Check sheet for the modelled part. Datum: model origin and axes. Units: mm. A direction names the side the tool comes from. Round coordinates to 2 decimals unless told otherwise and drop trailing zeros. Write each loop counter-clockwise with the first axis right and the second up, starting at its lowest first coordinate (ties: lowest second). Pieces come first, ordered by that corner, then holes. Notation, with made-up numbers: M 53.5,-4.75 L 76.5,-4.75 A11 ccw 76.5,-0.75 Z; hole C 22,41.25 d11. An arc over 180 degrees is marked long. Answer in a Markdown table with one row per item.
```python
from build123d import *

# Parameters (mm, degrees)
F0_W     = 20
F0_H     = 10
F1_DEPTH = 5
F2_W     = 5
F2_H     = 30
F3_DEPTH = 30
F4_W     = 20
F4_H     = 5
F5_DEPTH = 5
F6_R     = 5
F7_DEPTH = 5


with BuildPart() as f1:
    # F0 (on Front) → F1 (new body)
    with BuildSketch(Plane.XZ):
        Polygon((0, 100), (0, 0), (142, 0), (142, 100), (50.6040596026, 100), (50.6040596026, 121.4291932336), (20, 100), align=None)
        with Locations((30.5, 25)):
            Rectangle(F0_W, F0_H, mode=Mode.SUBTRACT)
        with Locations((71, 25)):
            Rectangle(F0_W, F0_H, mode=Mode.SUBTRACT)
        with Locations((111.5, 25)):
            Rectangle(F0_W, F0_H, mode=Mode.SUBTRACT)
        with Locations((30.5, 75)):
            Rectangle(F0_W, F0_H, mode=Mode.SUBTRACT)
        with Locations((71, 75)):
            Rectangle(F0_W, F0_H, mode=Mode.SUBTRACT)
        with Locations((111.5, 75)):
            Rectangle(F0_W, F0_H, mode=Mode.SUBTRACT)
    extrude(amount=F1_DEPTH)

    # F2 (on face) → F3 (join)
    with BuildSketch(Plane.XZ.offset(5)):
        with Locations((2.5, 40)):
            Rectangle(F2_W, F2_H)
        Polygon((50.6040596026, 121.4291932336), (20, 100), (28.7172339781, 100), (50.6040596026, 115.3253202898), align=None)
    extrude(amount=F3_DEPTH)

    # F4 (on face) → F5 (cut, through all)
    with BuildSketch(Plane.YZ.offset(5)):
        with Locations((-20, 47.5)):
            Rectangle(F4_W, F4_H)
        with Locations((-20, 32.5)):
            Rectangle(F4_W, F4_H)
    extrude(amount=-F5_DEPTH, mode=Mode.SUBTRACT)

    # F6 (on face) → F7 (cut, through all)
    with BuildSketch(Plane(origin=(-37.5369502908, 0, 53.608320737), x_dir=(0.8191520443, 0, 0.5735764364), z_dir=(0.5735764364, 0, -0.8191520443))):
        with Locations((93.7406845209, 20)):
            Circle(F6_R)
    extrude(amount=-F7_DEPTH, mode=Mode.SUBTRACT)


solid = f1.part
```
1. Section check A-A, the plane z = 76.5. Record the cut outline in (x, y).
Found:
| item | result |
|---|---|
| outline | M 0,-5 L 20.5,-5 L 20.5,0 L 0,0 Z; M 40.5,-5 L 61,-5 L 61,0 L 40.5,0 Z; M 81,-5 L 101.5,-5 L 101.5,0 L 81,0 Z; M 121.5,-5 L 142,-5 L 142,0 L 121.5,0 Z |
2. Access from +Z, -Z, +X, -X, +Y, -Y to the whole of each face (thin tool, end or side, straight path). Record for faces 4 (the face through (5, -20, 40)), 5 (the face through (50.604, -13, 118)), 6 (the face through (3, -10, 32)).
Found:
| item | result |
|---|---|
| face 4 | +Z, -Z, +X, -Y |
| face 5 | +Z, +X, +Y, -Y |
| face 6 | +X, -X |
3. Draft check along Z on faces 1 (the face through (0, -13, 40)), 2 (the face through (71, -2, 20)), 3 (the face through (2, -20, 25)). Enter one of: +Z half, -Z half, draft (parallel to the pull), parting line (faces both ways), or undercut.
Found:
| item | result |
|---|---|
| face 1 | draft |
| face 2 | undercut |
| face 3 | -Z half |
4. Scan lines: L1, parallel to X at y = -4.5, z = 21.5; L2, parallel to Y at x = 128, z = 46.5; L3, parallel to X at y = -20, z = 52.5. Record each from-to range of solid material in increasing order.
Found:
| item | result |
|---|---|
| L1 | x = 0 to 20.5, 40.5 to 61, 81 to 101.5, 121.5 to 142 |
| L2 | y = -5 to 0 |
| L3 | x = 0 to 5 |
5. Go/stop test with flat-tipped pins: pin 1 (4 mm diameter, centred on x = 2, y = -23, fed in from -Z); pin 2 (1 mm diameter, centred on x = 41, y = -16, fed in from +Z); pin 3 (5.5 mm diameter, centred on x = 2.5, y = -20, fed in from +Z). Record where each tip stops, or that it passes through.
Found:
| item | result |
|---|---|
| pin 1 | stops at z = 25 |
| pin 2 | stops at z = 115.05 |
| pin 3 | stops at z = 55 |
6. Section check D-D, the plane x = 95. Record the cut outline in (y, z).
Found:
| item | result |
|---|---|
| outline | M -5,0 L 0,0 L 0,100 L -5,100 Z |
7. Section check C-C, the plane z = 43. Record the cut outline in (x, y), and give its area (3 significant figures).
Found:
| item | result |
|---|---|
| outline | M 0,-35 L 5,-35 L 5,-5 L 142,-5 L 142,0 L 0,0 Z |
| area | 860 mm2 |
8. Section check B-B, the plane y = -28. Record the cut outline in (x, z).
Found:
| item | result |
|---|---|
| outline | M 0,25 L 5,25 L 5,30 L 0,30 Z; M 0,35 L 5,35 L 5,45 L 0,45 Z; M 0,50 L 5,50 L 5,55 L 0,55 Z; M 20,100 L 28.72,100 L 50.6,115.33 L 50.6,121.43 Z |
